Verification items for the finished model (mm, model axes). A direction names the side the tool comes from. Round coordinates to 2 decimals unless told otherwise and drop trailing zeros. Answer as a JSON object with one key per item and string values. Group by question number.
(1) Gauge pin test, flat ends, axial feed: pin 1 Ø1 at (x, y) = (40.5, -92) entering from -Z; pin 2 Ø19 at (x, y) = (60, 0) entering from +Z; pin 3 Ø1.5 at (y, z) = (7.5, 0) entering from +X; pin 4 Ø14 at (x, y) = (112.5, 0) entering from +Z. Record the tip position at first contact, or that the pin passes through.
(2) Draft check along X on faces 4 (the face through (59.605, -1.78, -26.175)), 5 (the face through (-21, 21, 12.038)), 6 (the face through (-131.627, 41.451, -8.158)). Enter one of: released by +X, released by -X, zero draft, split by the parting line, or undercut.
(3) Sectioned sample at A-A on y = -5.5. Count the separate pieces of the cut face and the enclosed holes in it, and give its area (3 significant figures).
(4) Scan lines: L1, parallel to Y at x = 0, z = -1.25; L2, parallel to Y at x = 56.25, z = -2; L3, parallel to Z at x = -26.5, y = -91. Record each from-to range of solid material in increasing order. Write a range as from..to.
(5) Set-up check for faces 1 (the face through (-43.545, 68.3, -25.004)), 2 (the face through (70.49, 0.46, -4.69)), 3 (the face through (66.87, 93.02, -7.77)): record each of +Z, -Z, +X, -X, +Y, -Y from which the full face is reachable in a straight line by a thin tool's end or side.
```python
from build123d import *

# Parameters (mm, degrees)
F2_R     = 11.5
F3_DEPTH = 81.001
F4_DEPTH = 28
F6_D     = 21
F6_DEPTH = 33
F6_TIP   = 6.3090364998
F7_D     = 10
F7_DEPTH = 18
F7_TIP   = 3.0043030951


with BuildPart() as f1:
    # F0 (on Front) → F1 (revolve)
    with BuildSketch(Plane.XZ):
        Polygon((-28, -37.9619441777), (-28, 12.0380558223), (-88, 12.0380558223), (-91.4641016151, 6.0380558223), (-138, 6.0380558223), (-138, -21.9619441777), (-81, -21.9619441777), (-81, -27.9619441777), (-35, -74.9619441777), (-14, -74.9619441777), (-14, -46.0448479464), align=None)
    revolve(axis=Axis((0, 0, -17.8461521864), (0, 0, -1)))

    # F2 (on face) → F3 (cut, through all)
    with BuildSketch(Plane.XY.offset(6.0380558223)):
        with Locations((-112.5, 0)):
            Circle(F2_R)
    extrude(amount=-F3_DEPTH, mode=Mode.SUBTRACT)

    # F2 (on face) → F4 (cut, through all)
    with BuildSketch(Plane.XY.offset(6.0380558223)):
        with Locations((-56.25, 97.4278579257)):
            Circle(F2_R)
        with Locations((56.25, 97.4278579257)):
            Circle(F2_R)
        with Locations((112.5, 0)):
            Circle(F2_R)
        with Locations((56.25, -97.4278579257)):
            Circle(F2_R)
        with Locations((-56.25, -97.4278579257)):
            Circle(F2_R)
    extrude(amount=-F4_DEPTH, mode=Mode.SUBTRACT)

    # F6
    with Locations(Plane.XY.offset(12.0380558223)):
        with Locations((-60, 0), (60, 0)):
            Hole(F6_D / 2, depth=F6_DEPTH)
            with Locations((0, 0, -(F6_DEPTH + F6_TIP / 2))):  # 118° drill point
                Cone(0, F6_D / 2, F6_TIP, mode=Mode.SUBTRACT)

    # F7
    with Locations(Plane.XY.offset(12.0380558223)):
        with Locations((0, 44), (0, -44)):
            Hole(F7_D / 2, depth=F7_DEPTH)
            with Locations((0, 0, -(F7_DEPTH + F7_TIP / 2))):  # 118° drill point
                Cone(0, F7_D / 2, F7_TIP, mode=Mode.SUBTRACT)


solid = f1.part
```
Computed values:
{
 "1": {"pin 1": "z = -21.96", "pin 2": "z = -21.56", "pin 3": "x = 137.83", "pin 4": "through"},
 "2": {"face 4": "undercut", "face 5": "zero draft", "face 6": "split by the parting line"},
 "3": {"separate pieces": "4", "enclosed holes": "0", "area": "9,000 mm2"},
 "4": {"L1": "-138..-49, -39..-28, 28..39, 49..138", "L2": "-126.02..-108.93, -85.93..-9.81, 9.81..85.93, 108.93..126.02", "L3": "-21.96..6.04"},
 "5": {"face 1": "-Z", "face 2": "+Z", "face 3": "+Z, -Z"}
}
